from build123d import *

# Parameters (mm, degrees)
F0_W     = 330.2
F0_H     = 101.6
F0_R     = 6.35
F0_R_2   = 3.175
F1_DEPTH = 12.7


with BuildPart() as f1:
    # F0 (on Right) → F1 (new body)
    with BuildSketch(Plane.YZ):
        with Locations((52.411457, 13.716)):
            Rectangle(F0_W, F0_H)
        with Locations((-99.988543, 26.416)):
            Circle(F0_R, mode=Mode.SUBTRACT)
        with Locations((39.711457, 13.716)):
            Circle(F0_R_2, mode=Mode.SUBTRACT)
    extrude(amount=F1_DEPTH)


solid = f1.part
Geometry check sheet. Reference: the model listing, model coordinates, mm. Round coordinates to 2 decimals unless told otherwise and drop trailing zeros.
Item 1: Material ranges on line 1 along Y through (x, z) = (9.5, 14); line 2 along Y through (x, z) = (10.75, 23.5), recorded low to high.
Determined:
line 1: y = -112.69 to 36.55, 42.87 to 217.51
line 2: y = -112.69 to -105.63, -94.35 to 217.51
Item 2: Mould release check, pull along Z, two halves, no side actions. Record for faces 1 (the face through (6, 50, -37.084)), 2 (the face through (12.7, 50, 14)), 3 (the face through (6.261, -106.332, 26.695)): +Z half, -Z half, draft (parallel to the pull), parting line (faces both ways), or undercut.
Determined:
face 1: -Z half
face 2: draft
face 3: undercut
Item 3: Go/stop test with a flat-tipped pin: pin 1 Ø7.5 at (y, z) = (-99.99, 26.42) entering from -X. Record where the tip stops, or that it passes through.
Determined:
pin 1: passes through
